```python
from build123d import *

# Parameters (mm, degrees)
F0_R     = 4.953
F1_DEPTH = 12.192
F2_DEPTH = 45.974
F4_DEPTH = 77.6025691706


with BuildPart() as f1:
    # F0 (on Top) → F1 (new body)
    with BuildSketch(Plane.XY):
        with BuildLine():
            ThreePointArc((0, 12.7), (3.7197438789, 3.7197438789), (12.7, 0))
            Line((12.7, 0), (50.8, 0))
            ThreePointArc((50.8, 0), (59.7802561211, 3.7197438789), (63.5, 12.7))
            Line((63.5, 12.7), (63.5, 76.2))
            ThreePointArc((63.5, 76.2), (59.7802561211, 85.1802561211), (50.8, 88.9))
            Line((50.8, 88.9), (12.7, 88.9))
            ThreePointArc((12.7, 88.9), (3.7197438789, 85.1802561211), (0, 76.2))
            Line((0, 76.2), (0, 12.7))
        make_face()
        with Locations((12.7, 12.7)):
            Circle(F0_R, mode=Mode.SUBTRACT)
        with Locations((50.8, 12.7)):
            Circle(F0_R, mode=Mode.SUBTRACT)
        Polygon((34.4043359374, 70.8815605479), (57.2736722661, 32.766), (30.0482718748, 16.4307597652), (7.178935546, 54.5463203131), align=None, mode=Mode.SUBTRACT)
        with BuildLine():
            ThreePointArc((8.5061583053, 73.5648717603), (8.452801422, 73.6517627193), (8.4012445439, 73.7397336468))
            ThreePointArc((8.4012445439, 73.7397336468), (11.4271148469, 80.9866452121), (17.653, 76.2))
            ThreePointArc((17.653, 76.2), (14.0711511744, 71.4405721503), (8.5061583053, 73.5648717603))
        make_face(mode=Mode.SUBTRACT)
        with Locations((50.8, 76.2)):
            Circle(F0_R, mode=Mode.SUBTRACT)
    extrude(amount=F1_DEPTH)

    # F0 (on Top) → F2 (join)
    with BuildSketch(Plane.XY):
        Polygon((30.0482718748, 16.4307597652), (57.2736722661, 32.766), (34.4043359374, 70.8815605479), (7.178935546, 54.5463203131), align=None)
    extrude(amount=F2_DEPTH)

    # F3 (on face) → F4 (cut, through all)
    with BuildSketch(Plane(origin=(0.7050897175, -1.1751495292, 0), x_dir=(0.8574929257, 0.5144957554, 0), z_dir=(0.5144957554, -0.8574929257, 0))):
        Polygon((62.6677367201, 45.974), (37.5217367201, 45.974), (46.9197367201, 32.004), (46.9197367201, 26.924), (53.2697367201, 26.924), (53.2697367201, 32.004), align=None)
    extrude(amount=-F4_DEPTH, mode=Mode.SUBTRACT)


solid = f1.part
```
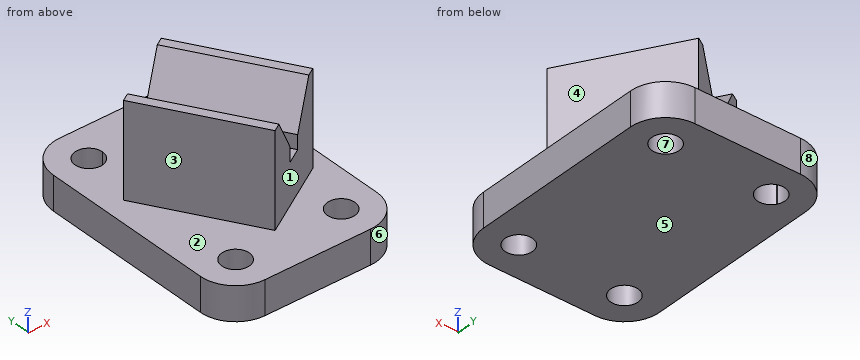
Input: part model. Units: mm. Frame: model coordinates. Face numbers are marked on the shaded views. A direction names the side the tool comes from. Round coordinates to 2 decimals unless told otherwise and drop trailing zeros. Loops run counter-clockwise (first coordinate to the right, second up) from the corner with the lowest first, then second, coordinate; pieces in that order, holes last.
1) Section query C-C on x = 36.5. Return the cut outline in (y, z).
Ans:
outline: (0, 0) - (88.9, 0) - (88.9, 12.19) - (67.39, 12.19) - (67.39, 45.97) - (60.97, 45.97) - (42.7, 32) - (42.7, 26.92) - (30.36, 26.92) - (30.36, 32) - (20.3, 39.7) - (20.3, 12.19) - (0, 12.19) - close
2) Pull-direction query (Y, two-part tool) for the marked faces 5, 6, 7 and 8; classes: released by +Y, released by -Y, zero draft, split by the parting line, or undercut.
Ans:
face 5: zero draft
face 6: released by -Y
face 7: undercut
face 8: released by +Y
3) Material intervals for line 1 (Y direction, x = 50.8, z = 5.75); line 2 (X direction, y = 76, z = 3); line 3 (Z direction, x = 6, y = 11.5), sorted ascending.
Ans:
line 1: y = 0 to 7.75, 17.65 to 71.25, 81.15 to 88.9
line 2: x = 0 to 7.75, 17.65 to 45.85, 55.75 to 63.5
line 3: z = 0 to 12.19
4) Set-up query: the marked faces 1, 2, 3 and 4. Return all of +Z, -Z, +X, -X, +Y, -Y with unobstructed straight access to the full face (end or side cutting, diameter ignored); none if empty.
Ans:
face 1: +Z, +X, -Y
face 2: +Z
face 3: +Z, -X, -Y
face 4: +Z, +X, +Y
5) Section query A-A on z = 6. Return the cut outline in (x, y), plus the area to 3 significant figures.
Ans:
outline: (0, 12.7) arc R12.7 ccw to (12.7, 0) - (50.8, 0) arc R12.7 ccw to (63.5, 12.7) - (63.5, 76.2) arc R12.7 ccw to (50.8, 88.9) - (12.7, 88.9) arc R12.7 ccw to (0, 76.2) - close; hole circle Ø9.91 at (12.7, 12.7); hole circle Ø9.91 at (12.7, 76.2); hole circle Ø9.91 at (50.8, 12.7); hole circle Ø9.91 at (50.8, 76.2)
area: 5,200 mm2
6) Section query B-B on z = 35. Return the cut outline in (x, y), plus the area to 3 significant figures.
Ans:
outline: (7.18, 54.55) - (30.05, 16.43) - (39.21, 21.93) - (16.34, 60.04) - close; (25.24, 65.38) - (48.11, 27.27) - (57.27, 32.77) - (34.4, 70.88) - close
area: 950 mm2
7) Pin query (flat end, axial travel): pin 1 (16 mm diameter, centred on x = 12.7, y = 76.2, fed in from -Z); pin 2 (8 mm diameter, centred on x = 50.8, y = 76.2, fed in from +Z); pin 3 (6 mm diameter, centred on x = 17.5, z = 38.5, fed in from -Y); pin 4 (8 mm diameter, centred on x = 37, y = 23, fed in from +Z). Return the tip coordinate at first contact, or that it passes through.
Ans:
pin 1: stops at z = 0
pin 2: passes through
pin 3: stops at y = 32.34
pin 4: stops at z = 42.94
8) Section query D-D on y = 35. Return the cut outline in (x, z), plus the area to 3 significant figures.
Ans:
outline: (0, 0) - (63.5, 0) - (63.5, 12.19) - (55.93, 12.19) - (55.93, 45.97) - (52.08, 45.97) - (41.12, 32) - (41.12, 26.92) - (33.72, 26.92) - (33.72, 32) - (22.76, 45.97) - (18.91, 45.97) - (18.91, 12.19) - (0, 12.19) - close
area: 1,730 mm2
